Answer from the drawing. Dimensions are ordinates in mm from the lowest x, y and z of the part. A direction names the side the tool comes from. Give positions to 0.01 mm unless a question says otherwise; leave off trailing zeros. Write each loop counter-clockwise with the first axis right and the second up, starting at its lowest first coordinate (ties: lowest second). Pieces come first, ordered by that corner, then holes.
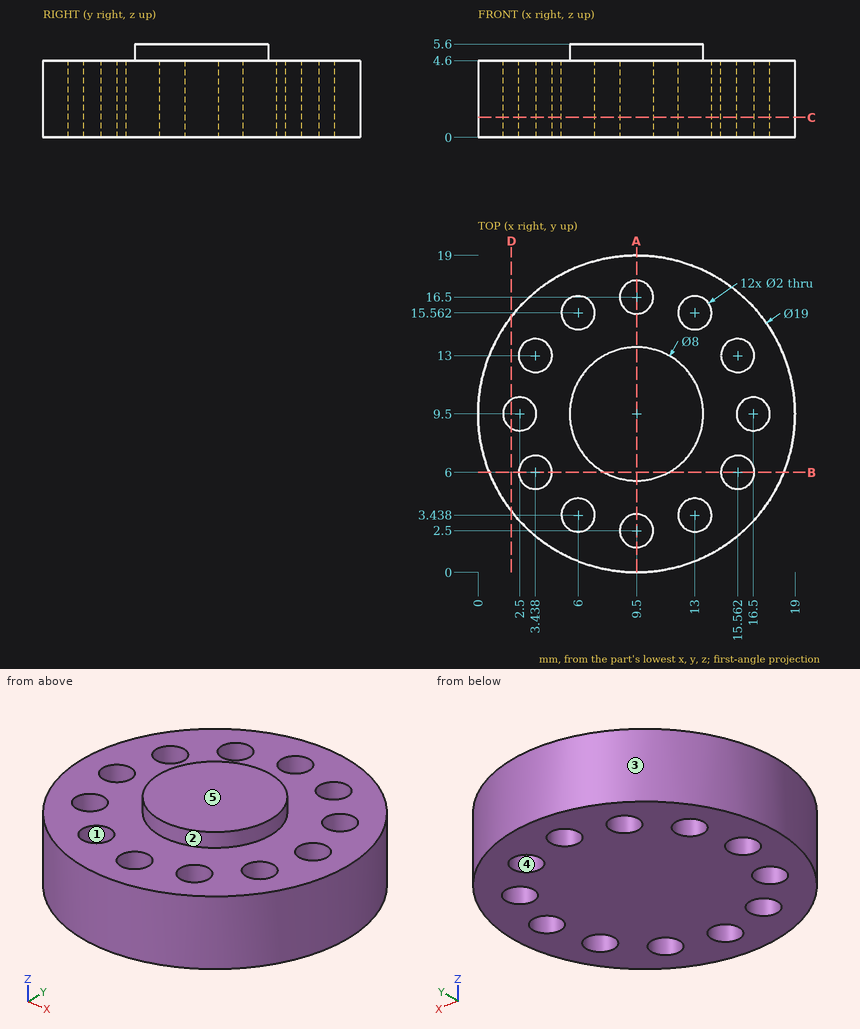
Item 1: Section A-A (x = 9.5) is taken. Write down the section's boundary in (y, z).
Result set:
outline: (0, 0) - (1.5, 0) - (1.5, 4.6) - (0, 4.6) - close; (3.5, 0) - (15.5, 0) - (15.5, 4.6) - (13.5, 4.6) - (13.5, 5.6) - (5.5, 5.6) - (5.5, 4.6) - (3.5, 4.6) - close; (17.5, 0) - (19, 0) - (19, 4.6) - (17.5, 4.6) - close
Item 2: Each of these flat-tipped pins is pushed along its axis until it touches: pin 1 Ø3 at (x, y) = (6, 3.44) entering from +Z; pin 2 Ø2 at (x, z) = (5, 2.5) entering from -Y; pin 3 Ø1.8 at (x, y) = (16.5, 9.5) entering from +Z; pin 4 Ø1 at (y, z) = (13.5, 5) entering from -X. Where does it stop, or does it pass through?
Result set:
pin 1: stops at z = 4.6
pin 2: stops at y = 0.67
pin 3: passes through
pin 4: stops at x = 0.75
Item 3: Which of the six approach directions +Z, -Z, +X, -X, +Y, -Y give full straight-line access (tool end or side, diameter ignored) to the marked faces 1 and 2?
Result set:
face 1: +Z, -Z
face 2: +Z
Item 4: Section C-C (z = 1.2) is taken. Give the number of separate pieces and of enclosed holes in the cut face, and give its area (3 significant figures).
Result set:
separate pieces: 1
enclosed holes: 12
area: 246 mm2
Item 5: Section D-D (x = 2) is taken. Write down the section's boundary in (y, z).
Result set:
outline: (3.67, 0) - (8.63, 0) - (8.63, 4.6) - (3.67, 4.6) - close; (10.37, 0) - (15.33, 0) - (15.33, 4.6) - (10.37, 4.6) - close
Item 6: Find the intervals of material crossed by line 1 along X through (y, z) = (9.5, 1.7); line 2 along X through (y, z) = (6.25, 1.85); line 3 along Y through (x, z) = (13.75, 3.6), in increasing order.
Result set:
line 1: x = 0 to 1.5, 3.5 to 15.5, 17.5 to 19
line 2: x = 0.57 to 2.47, 4.41 to 14.59, 16.53 to 18.43
line 3: y = 1 to 2.78, 4.1 to 14.9, 16.22 to 18
Item 7: Determine the mould class of the marked faces 3, 4 and 5 for opening direction X: pulls with the +X half, pulls with the -X half, needs draft (parallel to the pull), parting line crosses it, or undercut.
Result set:
face 3: parting line crosses it
face 4: undercut
face 5: needs draft
Item 8: Section B-B (y = 6) is taken. Write down the section's boundary in (x, z), and give its area (3 significant figures).
Result set:
outline: (0.67, 0) - (2.44, 0) - (2.44, 4.6) - (0.67, 4.6) - close; (4.44, 0) - (14.56, 0) - (14.56, 4.6) - (11.44, 4.6) - (11.44, 5.6) - (7.56, 5.6) - (7.56, 4.6) - (4.44, 4.6) - close; (16.56, 0) - (18.33, 0) - (18.33, 4.6) - (16.56, 4.6) - close
area: 66.7 mm2
